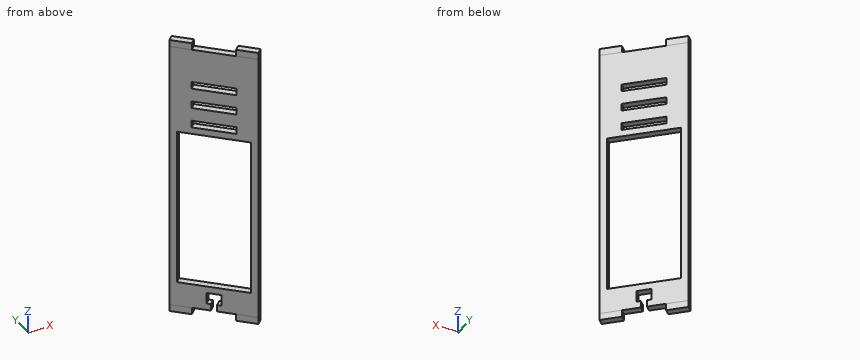
from build123d import *

# Parameters (mm, degrees)
BOSS_EXTRUDE1_DEPTH = 200
SKETCH3_W           = 15
SKETCH3_H           = 5
BOSS_EXTRUDE2_DEPTH = 5
SKETCH4_W           = 30.2
SKETCH4_H           = 5.2
CUT_EXTRUDE1_DEPTH  = 5
SKETCH5_W           = 4.2
SKETCH5_H           = 5
CUT_EXTRUDE2_DEPTH  = 10
SKETCH6_W           = 50
SKETCH6_H           = 116.6
CUT_EXTRUDE3_DEPTH  = 10


with BuildPart() as part:
    # Sketch1 → Boss-Extrude1 (new body)
    with BuildSketch(Plane.XY):
        Polygon((34.899243254, 77.987452967), (77.573371526, 35.810222425), (81.088140738, 39.366399781), (38.414012466, 81.543630323), align=None)
    extrude(amount=BOSS_EXTRUDE1_DEPTH)

    # Sketch3 → Boss-Extrude2 (add)
    with BuildSketch(Plane(origin=(56.23630739, 56.898837696, 0), x_dir=(0.711235471, -0.702953842, 0), z_dir=(-0.702953842, -0.711235471, 0))):
        with Locations((-22.5, 202.5)):
            Rectangle(SKETCH3_W, SKETCH3_H)
        with Locations((22.5, 202.5)):
            Rectangle(SKETCH3_W, SKETCH3_H)
        with Locations((22.5, -2.5)):
            Rectangle(SKETCH3_W, SKETCH3_H)
        with Locations((-22.5, -2.5)):
            Rectangle(SKETCH3_W, SKETCH3_H)
    extrude(amount=-BOSS_EXTRUDE2_DEPTH)

    # Sketch4 → Cut-Extrude1 (cut)
    with BuildSketch(Plane(origin=(56.23630739, 56.898837696, 0), x_dir=(0.711235471, -0.702953842, 0), z_dir=(-0.702953842, -0.711235471, 0))):
        with Locations((0, 172.4)):
            Rectangle(SKETCH4_W, SKETCH4_H)
        with Locations((0, 157.4)):
            Rectangle(SKETCH4_W, SKETCH4_H)
        with Locations((0, 142.4)):
            Rectangle(SKETCH4_W, SKETCH4_H)
    extrude(amount=-CUT_EXTRUDE1_DEPTH, mode=Mode.SUBTRACT)

    # Sketch5 → Cut-Extrude2 (cut)
    with BuildSketch(Plane(origin=(59.751076602, 60.455015052, 0), x_dir=(0.711235471, -0.702953842, 0), z_dir=(0.702953842, 0.711235471, 0))):
        Polygon((2.1, -5), (-2.1, -5), (-5, -5), (-5, -13.2), (5, -13.2), (5, -5), align=None)
        with Locations((0, -2.5)):
            Rectangle(SKETCH5_W, SKETCH5_H)
    extrude(amount=-CUT_EXTRUDE2_DEPTH, mode=Mode.SUBTRACT)

    # Sketch6 → Cut-Extrude3 (cut)
    with BuildSketch(Plane(origin=(59.751076602, 60.455015052, 0), x_dir=(0.711235471, -0.702953842, 0), z_dir=(0.702953842, 0.711235471, 0))):
        with Locations((0, -76.5)):
            Rectangle(SKETCH6_W, SKETCH6_H)
    extrude(amount=-CUT_EXTRUDE3_DEPTH, mode=Mode.SUBTRACT)


solid = part.part
Check sheet for the modelled part. Datum: model origin and axes. Units: mm. Give positions to 0.01 mm unless a question says otherwise; leave off trailing zeros. Write each loop counter-clockwise with the first axis right and the second up, starting at its lowest first coordinate (ties: lowest second). Pieces come first, ordered by that corner, then holes. Notation, with made-up numbers: (82.25, 39.5) -> (97.25, 39.5) arc R11 ccw to (97.25, 44.5) -> close; hole circle Ø3 at (51.5, -20). An arc over 180 degrees is marked (long way). Write item = value, one per line.
Item 1: Sectioned sample at A-A on z = 65.5. Record the boundary of the cut face in (x, y) (3 decimals).
Output:
outline = (34.899, 77.987) -> (38.455, 74.473) -> (41.97, 78.029) -> (38.414, 81.544) -> close; (74.017, 39.325) -> (77.573, 35.81) -> (81.088, 39.366) -> (77.532, 42.881) -> close
Item 2: Sectioned sample at B-B on z = 179. Record the boundary of the cut face in (x, y), and give its area (3 significant figures).
Output:
outline = (34.9, 77.99) -> (77.57, 35.81) -> (81.09, 39.37) -> (38.41, 81.54) -> close
area = 300 mm^2
Item 3: Gauge pin test, flat ends, axial feed: pin 1 (1.5 mm diameter, centred on x = 72.5, z = 60, fed in from -Y); pin 2 (7.5 mm diameter, centred on x = 58.5, y = 59, fed in from +Z); pin 3 (20 mm diameter, centred on x = 62, y = 60.5, fed in from -Z); pin 4 (3 mm diameter, centred on x = 59.5, y = 60.5, fed in from -Z). Record the tip position at first contact, or that the pin passes through.
Output:
pin_1 = through
pin_2 = 200
pin_3 = 0
pin_4 = 13.2
Item 4: Scan lines: probe 1 along Z at (x, y) = (54.5, 62); probe 2 along Z at (x, y) = (57, 57); probe 3 along Z at (x, y) = (44.5, 69.5). Record each from-to range of solid material in increasing order. Write a range as from..to.
Output:
probe_1 = 0..5, 13.2..18.2, 134.8..139.8, 145..154.8, 160..169.8, 175..200
probe_2 = 13.2..18.2, 134.8..139.8, 145..154.8, 160..169.8, 175..200
probe_3 = -5..18.2, 134.8..205
